Geometry check sheet. Reference: the model listing, model coordinates, mm. A direction names the side the tool comes from. Round coordinates to 2 decimals unless told otherwise and drop trailing zeros. Order: outer loops, then holes, each group sorted by start corner. A loop starts at its lowest first (then second) coordinate and runs counter-clockwise, first axis right, second up.
```python
from build123d import *

# Parameters (mm, degrees)
SKETCH_W        = 46
SKETCH_H        = 46
PAD_DEPTH       = 40
SKETCH001_R     = 17
POCKET_DEPTH    = 40.001
SKETCH002_R     = 3
POCKET001_DEPTH = 20


with BuildPart() as part:
    # Sketch → Pad (new body)
    with BuildSketch(Plane.XY):
        Rectangle(SKETCH_W, SKETCH_H)
    extrude(amount=PAD_DEPTH)

    # Sketch001 (on Face6 of Pad) → Pocket (cut, through all)
    with BuildSketch(Plane.XY.offset(40)):
        Circle(SKETCH001_R)
    extrude(amount=-POCKET_DEPTH, mode=Mode.SUBTRACT)

    # Sketch002 (on Face5 of Pocket) → Pocket001 (cut)
    with BuildSketch(Plane.XY.offset(40)):
        with Locations((16.5, 20.75)):
            Circle(SKETCH002_R)
        with Locations((-16.5, 20.75)):
            Circle(SKETCH002_R)
        with Locations((-16.5, -20.75)):
            Circle(SKETCH002_R)
        with Locations((16.5, -20.75)):
            Circle(SKETCH002_R)
    extrude(amount=-POCKET001_DEPTH, mode=Mode.SUBTRACT)


solid = part.part
```
(1) Draft check along X on faces 3 (the cylindrical face through (-16.6, 17.75, 30.14)), 4 (the flat face through (23, 0, 20)), 5 (the flat face through (-23, 0, 20)), 6 (the flat face through (-16, -10, 40)). Enter one of: released by +X, released by -X, zero draft, split by the parting line, or undercut.
Returned:
face 3: undercut
face 4: released by +X
face 5: released by -X
face 6: zero draft
(2) Sectioned sample at D-D, the plane z = 16. Record the cut outline in (x, y).
Returned:
outline: (-23, -23) - (23, -23) - (23, 23) - (-23, 23) - close; hole circle Ø34 at (0, 0)
(3) Sectioned sample at C-C, the plane y = 20.75. Record the cut outline in (x, z).
Returned:
outline: (-23, 0) - (23, 0) - (23, 40) - (19.5, 40) - (19.5, 20) - (13.5, 20) - (13.5, 40) - (-13.5, 40) - (-13.5, 20) - (-19.5, 20) - (-19.5, 40) - (-23, 40) - close
(4) Set-up check for faces 1 (the flat face through (0, 23, 20)), 2 (the cylindrical face through (-16.4, -17.75, 30.14)): record each of +Z, -Z, +X, -X, +Y, -Y from which the full face is reachable in a straight line by a thin tool's end or side.
Returned:
face 1: +Z, -Z, +X, -X, +Y
face 2: +Z
(5) Sectioned sample at A-A, the plane y = 0. Record the cut outline in (x, z).
Returned:
outline: (-23, 0) - (-17, 0) - (-17, 40) - (-23, 40) - close; (17, 0) - (23, 0) - (23, 40) - (17, 40) - close
(6) Material ranges on line 1 (X direction, y = -20.75, z = 28); line 2 (Y direction, x = -1.5, z = 20.5); line 3 (X direction, y = -20, z = 25), recorded low to high.
Returned:
line 1: x = -23 to -19.5, -13.5 to 13.5, 19.5 to 23
line 2: y = -23 to -16.93, 16.93 to 23
line 3: x = -23 to -19.4, -13.6 to 13.6, 19.4 to 23
(7) Depth check by flat-ended pin: P1, Ø20.5, axis at x = 0, y = 0, coming from the -Z side; P2, Ø2.5, axis at x = 18, y = -21, coming from the +Z side. Enter the tip coordinate at first touch or a pass-through.
Returned:
P1: passes through
P2: stops at z = 20
